The listing builds one solid part. Answer for the finished solid, in the listing's coordinates (mm). Coordinates: 2 decimals unless noted, no trailing zeros. Order: outer loops, then holes, each group sorted by start corner. A loop starts at its lowest first (then second) coordinate and runs counter-clockwise, first axis right, second up.
```python
from build123d import *

# Parameters (mm, degrees)
F0_R     = 384.4222137889
F1_DEPTH = 60
F1_TAPER = 15


with BuildPart() as f1:
    # F0 (on Front) → F1 (new body, symmetric)
    with BuildSketch(Plane.XZ):
        Circle(F0_R)
        with BuildLine():
            ThreePointArc((-306.5168000492, -122.798580153), (-324.2251435162, -62.5307629242), (-330.2, 0))
            ThreePointArc((-330.2, 0), (-325.6867721675, 54.4074115828), (-312.2704637484, 107.3275242906))
            ThreePointArc((-312.2704637484, 107.3275242906), (-284.6368182454, 167.37359917), (-245.597160306, 220.7126522191))
            ThreePointArc((-245.597160306, 220.7126522191), (-189.128113572, 270.670642399), (-122.798580153, 306.5168000492))
            ThreePointArc((-122.798580153, 306.5168000492), (-62.5307629242, 324.2251435162), (0, 330.2))
            ThreePointArc((0, 330.2), (70.9592964928, 322.4853767867), (138.6028798667, 299.701988136))
            ThreePointArc((138.6028798667, 299.701988136), (205.1525193234, 258.7363210205), (260.2112729594, 203.2784627668))
            ThreePointArc((260.2112729594, 203.2784627668), (286.2069706705, 164.6742540278), (306.5168000492, 122.798580153))
            ThreePointArc((306.5168000492, 122.798580153), (324.2251435162, 62.5307629242), (330.2, 0))
            ThreePointArc((330.2, 0), (325.4397731908, -55.8658574223), (311.2963414565, -110.1209689195))
            ThreePointArc((311.2963414565, -110.1209689195), (283.8841721197, -168.6470184139), (245.597160306, -220.7126522191))
            ThreePointArc((245.597160306, -220.7126522191), (189.128113572, -270.670642399), (122.798580153, -306.5168000492))
            ThreePointArc((122.798580153, -306.5168000492), (62.5307629242, -324.2251435162), (0, -330.2))
            ThreePointArc((0, -330.2), (-78.1374463344, -320.8217253871), (-151.8364043025, -293.2196213225))
            ThreePointArc((-151.8364043025, -293.2196213225), (-210.8747853225, -254.0942048044), (-260.2112729594, -203.2784627668))
            ThreePointArc((-260.2112729594, -203.2784627668), (-286.2069706705, -164.6742540278), (-306.5168000492, -122.798580153))
        make_face(mode=Mode.SUBTRACT)
    extrude(amount=F1_DEPTH, both=True, taper=F1_TAPER)


solid = f1.part
```
(1) Each of these flat-tipped pins is pushed along its axis until it touches: pin 1 Ø1.5 at (x, y) = (264.5, -45.5) entering from +Z; pin 2 Ø2 at (x, y) = (-231, -5) entering from +Z; pin 3 Ø6 at (x, y) = (-122.5, 0.5) entering from +Z. Where does it stop, or does it pass through?
(2) Consider line 1 (Z direction, x = 223, y = -37); line 2 (Z direction, x = -212, y = -11); line 3 (X direction, y = -37.5, z = 168.5). Determine where each line is inside the solid, lowest interval first.
(3) Find section A-A (y = 16). Write down the section's boundary in (x, z).
Findings below:
1. pin 1: stops at z = 262.71
1. pin 2: stops at z = 306.42
1. pin 3: stops at z = 365.36
2. line 1: z = -300.88 to -256.8, 256.8 to 300.88
2. line 2: z = -317.14 to -256.99, 256.99 to 317.14
2. line 3: x = -334.31 to -295.6, 295.6 to 334.31
3. outline: circle Ø760.27 at (0, 0); hole circle Ø668.97 at (0, 0)
